from build123d import *

# Parameters (mm, degrees)
ESQUISSE1_R             = 25.5
BOSS_EXTRU_1_DEPTH      = 18
ENL_V_MAT_EXTRU_2_DEPTH = 10
ENL_V_MAT_EXTRU_4_DEPTH = 5
CONG_1_R                = 0.3


with BuildPart() as part:
    # Esquisse1 → Boss.-Extru.1 (new body)
    with BuildSketch(Plane.XY):
        Circle(ESQUISSE1_R)
    extrude(amount=BOSS_EXTRU_1_DEPTH)

    # Esquisse2 → Enlèv. mat.-Extru.2 (cut)
    with BuildSketch(Plane.XY.offset(18)):
        with BuildLine():
            Line((1.322875656, 1.5), (-1.322875656, 1.5))
            ThreePointArc((-1.322875656, 1.5), (0, -2), (1.322875656, 1.5))
        make_face()
    extrude(amount=-ENL_V_MAT_EXTRU_2_DEPTH, mode=Mode.SUBTRACT)

    # Esquisse3 → Enlèv. mat.-Extru.4 (cut)
    with BuildSketch(Plane(origin=(0, 0, 0), x_dir=(-1, 0, 0), z_dir=(0, 0, -1))):
        with BuildLine():
            ThreePointArc((1.5, 3.708324452), (2.828574751, 2.828574751), (3.708324452, 1.5))
            Line((3.708324452, 1.5), (23.953079134, 1.5))
            ThreePointArc((23.953079134, 1.5), (16.970562748, 16.970562748), (1.5, 23.953079134))
            Line((1.5, 23.953079134), (1.5, 3.708324452))
        make_face()
        with BuildLine():
            Line((-23.953079134, 1.5), (-3.708324452, 1.5))
            ThreePointArc((-3.708324452, 1.5), (-2.828574751, 2.828574751), (-1.5, 3.708324452))
            Line((-1.5, 3.708324452), (-1.5, 23.953079134))
            ThreePointArc((-1.5, 23.953079134), (-16.970562748, 16.970562748), (-23.953079134, 1.5))
        make_face()
        with BuildLine():
            Line((-1.5, -23.953079134), (-1.5, -3.708324452))
            ThreePointArc((-1.5, -3.708324452), (-2.828574751, -2.828574751), (-3.708324452, -1.5))
            Line((-3.708324452, -1.5), (-23.953079134, -1.5))
            ThreePointArc((-23.953079134, -1.5), (-16.970562748, -16.970562748), (-1.5, -23.953079134))
        make_face()
        with BuildLine():
            ThreePointArc((3.708324452, -1.5), (2.828574751, -2.828574751), (1.5, -3.708324452))
            Line((1.5, -3.708324452), (1.5, -23.953079134))
            ThreePointArc((1.5, -23.953079134), (16.970562748, -16.970562748), (23.953079134, -1.5))
            Line((23.953079134, -1.5), (3.708324452, -1.5))
        make_face()
    extrude(amount=-ENL_V_MAT_EXTRU_4_DEPTH, mode=Mode.SUBTRACT)

    # Congé1
    cong_1_edges = [part.edges().sort_by_distance(p)[0] for p in [
        (-25.5, 0, 0),
        (-25.5, 0, 18),
        (0, -2, 18),
        (0, 1.5, 18),
    ]]
    fillet(cong_1_edges, radius=CONG_1_R)


solid = part.part
The model under review builds one solid part; all positions refer to its coordinate system, in mm. A direction names the side the tool comes from. Give positions to 0.01 mm unless a question says otherwise; leave off trailing zeros. Loops run counter-clockwise (first coordinate to the right, second up) from the corner with the lowest first, then second, coordinate; pieces in that order, holes last. Notation, with made-up numbers: (31, 43) -> (41, 43) arc R28 ccw to (41, 74) -> close; hole circle Ø1 at (3, 59.25). An arc over 180 degrees is marked (long way). Answer as a JSON object with one key per item and string values. Group by question number.
Q1. Draft analysis for pull direction Y (two halves, no side actions). For faces 1 (the flat face through (1.5, -14, 2)), 2 (the flat face through (-10, -10, 5)), 3 (the cylindrical face through (-5.5, -24.9, 8.9)), state which applies: pulls with the +Y half, pulls with the -Y half, needs draft (parallel to the pull), parting line crosses it, or undercut.
Q2. Take a section at D-D (z = 6.25). Write out the cut boundary in (x, y).
Q3. Take a section at B-B (x = 0). Write out the cut boundary in (y, z), plus the area to 3 significant figures.
Q4. Insertion check: pin 1 (2 mm diameter, centred on x = 0, z = 13.5, fed in from -Y); pin 2 (2.5 mm diameter, centred on y = -13.5, z = 2, fed in from -X); pin 3 (2.5 mm diameter, centred on x = 11.5, z = 3, fed in from -Y). Each pin has a flat end and moves straight along its axis. Give the tip position at first contact, or say it passes through.
Q5. Tool access review of faces 4 (the cylindrical face through (0, -2, 13)), 5 (the cylindrical face through (-17.14, 16.8, 2.46)): name each direction out of +Z, -Z, +X, -X, +Y, -Y from which nothing blocks a thin tool from reaching the whole face with its end or side.
Q6. Take a section at A-A (z = 1.5). Write out the cut boundary in (x, y), plus the area to 3 significant figures.
Q7. Wall thickness on line 1 along Y through (x, z) = (0, 11); line 2 along Z through (x, y) = (8, -22.5); line 3 along Z through (x, y) = (19.5, 16): over which ranges is each line inside the solid? List them lowest first.
Q8. Take a section at C-C (z = 15). Write out the cut boundary in (x, y).
Answer below:
{
 "1": {"face 1": "undercut", "face 2": "undercut", "face 3": "parting line crosses it"},
 "2": {"outline": "circle Ø51 at (0, 0)"},
 "3": {"outline": "(-25.5, 0.3) arc R0.3 ccw to (-25.2, 0) -> (25.2, 0) arc R0.3 ccw to (25.5, 0.3) -> (25.5, 17.7) arc R0.3 ccw to (25.2, 18) -> (1.8, 18) arc R0.3 ccw to (1.5, 17.7) -> (1.5, 8) -> (-2, 8) -> (-2, 17.7) arc R0.3 ccw to (-2.3, 18) -> (-25.2, 18) arc R0.3 ccw to (-25.5, 17.7) -> close", "area": "883 mm2"},
 "4": {"pin 1": "stops at y = -25.5", "pin 2": "stops at x = -22.36", "pin 3": "stops at y = -23.35"},
 "5": {"face 4": "+Z", "face 5": "-Z"},
 "6": {"outline": "circle Ø51 at (0, 0); hole (-23.95, -1.5) arc R24 ccw to (-1.5, -23.95) -> (-1.5, -3.71) arc R4 cw to (-3.71, -1.5) -> close; hole (-23.95, 1.5) -> (-3.71, 1.5) arc R4 cw to (-1.5, 3.71) -> (-1.5, 23.95) arc R24 ccw to start; hole (1.5, -23.95) arc R24 ccw to (23.95, -1.5) -> (3.71, -1.5) arc R4 cw to (1.5, -3.71) -> close; hole (1.5, 3.71) arc R4 cw to (3.71, 1.5) -> (23.95, 1.5) arc R24 ccw to (1.5, 23.95) -> close", "area": "524 mm2"},
 "7": {"line 1": "y = -25.5 to -2, 1.5 to 25.5", "line 2": "z = 5 to 18", "line 3": "z = 0 to 18"},
 "8": {"outline": "circle Ø51 at (0, 0); hole (-1.32, 1.5) arc R2 ccw (long way) to (1.32, 1.5) -> close"}
}
